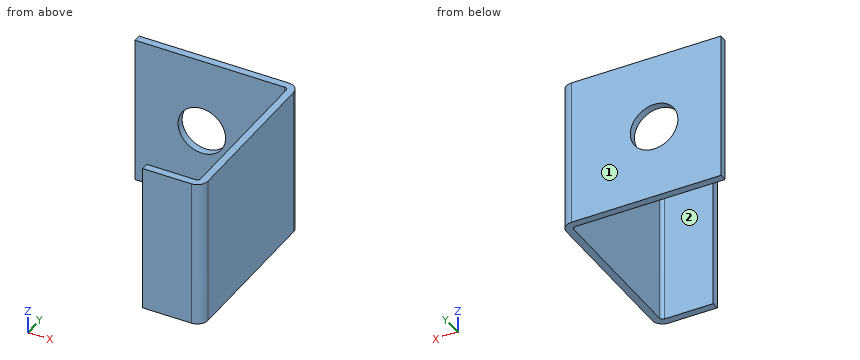
```python
from build123d import *

# Parameters (mm, degrees)
SKETCH1_W                     = 32.7025
SKETCH1_H                     = 31.75
SKETCH1_R                     = 5.08
HV_FUSE_BASE_DEPTH            = 1.5875
FUSE_TO_STACK_STRIP_W         = 7.8232
FUSE_TO_STACK_STRIP_H         = 1.5875
FUSE_TO_STACK_STRIP_CUT_DEPTH = 31.75
FUSE_TO_STACK_DEPTH           = 31.75
STACK_BASE_STRIP_W            = 7.8232
STACK_BASE_STRIP_H            = 1.5875
STACK_BASE_STRIP_CUT_DEPTH    = 31.75
STACK_BASE_DEPTH              = 31.75


# Sheet-metal steps are written as plain solids
with BuildPart() as part:
    # Sketch1 → HV Fuse Base (new body)
    with BuildSketch(Plane(origin=(0, 0, 0), x_dir=(1, 0, 0), z_dir=(0, 1, 0))):
        with Locations((16.35125, -15.875)):
            Rectangle(SKETCH1_W, SKETCH1_H)
        with Locations(Location((14.2875, -15.875, 0), (0, 0, 270))):
            Circle(SKETCH1_R, mode=Mode.SUBTRACT)
    extrude(amount=-HV_FUSE_BASE_DEPTH)

    # Fuse to Stack strip (across the edge) → Fuse to Stack strip cut (cut)
    with BuildSketch(Plane(origin=(32.7025, -1.5875, 0), x_dir=(-1, 0, 0), z_dir=(0, 0, 1))):
        with Locations((-3.175, -0.79375)):
            Rectangle(FUSE_TO_STACK_STRIP_W, FUSE_TO_STACK_STRIP_H)
    extrude(amount=FUSE_TO_STACK_STRIP_CUT_DEPTH, mode=Mode.SUBTRACT)

    # Fuse to Stack section (across the edge) → Fuse to Stack (add)
    with BuildSketch(Plane(origin=(32.7025, -1.5875, 0), x_dir=(-1, 0, 0), z_dir=(0, 0, 1))):
        with BuildLine():
            Line((-1.5875, 0.7366), (-1.5875, 36.22802))
            Line((-1.5875, 36.22802), (0, 36.22802))
            Line((0, 36.22802), (0, 0.7366))
            ThreePointArc((0, 0.7366), (0.215745145, 0.215745145), (0.7366, 0))
            Line((0.7366, 0), (0.7366, -1.5875))
            ThreePointArc((0.7366, -1.5875), (-0.90678687, -0.90678687), (-1.5875, 0.7366))
        make_face()
    extrude(amount=FUSE_TO_STACK_DEPTH)

    # Stack Base strip (across the edge) → Stack Base strip cut (cut)
    with BuildSketch(Plane(origin=(32.7025, -37.81552, 0), x_dir=(0, 1, 0), z_dir=(0, 0, 1))):
        with Locations((-1.5875, -0.79375)):
            Rectangle(STACK_BASE_STRIP_W, STACK_BASE_STRIP_H)
    extrude(amount=STACK_BASE_STRIP_CUT_DEPTH, mode=Mode.SUBTRACT)

    # Stack Base section (across the edge) → Stack Base (add)
    with BuildSketch(Plane(origin=(32.7025, -37.81552, 0), x_dir=(0, 1, 0), z_dir=(0, 0, 1))):
        with BuildLine():
            Line((0, 0.7366), (0, 11.1125))
            Line((0, 11.1125), (1.5875, 11.1125))
            Line((1.5875, 11.1125), (1.5875, 0.7366))
            ThreePointArc((1.5875, 0.7366), (1.803245145, 0.215745145), (2.3241, 0))
            Line((2.3241, 0), (2.3241, -1.5875))
            ThreePointArc((2.3241, -1.5875), (0.68071313, -0.90678687), (0, 0.7366))
        make_face()
    extrude(amount=STACK_BASE_DEPTH)


solid = part.part
```
Verification items for the finished model (mm, model axes). Face numbers are marked on the shaded views. A direction names the side the tool comes from. Give positions to 0.01 mm unless a question says otherwise; leave off trailing zeros. Order: outer loops, then holes, each group sorted by start corner. A loop starts at its lowest first (then second) coordinate and runs counter-clockwise, first axis right, second up. Notation, with made-up numbers: M -4,10.25 L 27,10.25 A14 ccw 27,15.25 Z; hole C 33.25,24.5 d3. An arc over 180 degrees is marked long. Return JSON: item names as keys, results as strings. Group by question number.
1) Go/stop test with flat-tipped pins: pin 1 Ø1.5 at (y, z) = (-12.5, 5.5) entering from -X; pin 2 Ø6 at (x, y) = (28, -33) entering from +Z; pin 3 Ø11.5 at (x, z) = (14.29, 15.88) entering from -Y; pin 4 Ø1.7 at (y, z) = (-37, 13.5) entering from -X. Record where each tip stops, or that it passes through.
2) Section check B-B on z = 24. Record the cut outline in (x, y), and give its area (3 significant figures).
3) Access from +Z, -Z, +X, -X, +Y, -Y to the whole of each face (thin tool, end or side, straight path). Record for the marked faces 1 and 2.
4) Section check C-C on x = 13. Record the cut outline in (y, z), and give its area (3 significant figures).
5) Section check A-A on x = 29.5. Record the cut outline in (y, z), and give its area (3 significant figures).
6) Scan lines: line 1 (Y direction, x = 23, z = 14); line 2 (Y direction, x = 4.5, z = 18.5); line 3 (X direction, y = -30, z = 21). Record each from-to range of solid material in increasing order.
7) Section check D-D on z = 20. Record the cut outline in (x, y), and give its area (3 significant figures).
Answer block:
{
 "1": {"pin 1": "stops at x = 32.7", "pin 2": "passes through", "pin 3": "stops at y = -1.59", "pin 4": "stops at x = 21.59"},
 "2": {"outline": "M 0,-1.59 L 31.97,-1.59 A0.74 cw 32.7,-2.32 L 32.7,-35.49 A0.74 cw 31.97,-36.23 L 21.59,-36.23 L 21.59,-37.82 L 31.97,-37.82 A2.32 ccw 34.29,-35.49 L 34.29,-2.32 A2.32 ccw 31.97,0 L 0,0 Z", "area": "128 mm^2"},
 "3": {"face 1": "+Z, -Z, +X, -X, +Y", "face 2": "+Z, -Z, -X"},
 "4": {"outline": "M -1.59,0 L 0,0 L 0,10.96 L -1.59,10.96 Z; M -1.59,20.79 L 0,20.79 L 0,31.75 L -1.59,31.75 Z", "area": "34.8 mm^2"},
 "5": {"outline": "M -37.82,0 L -36.23,0 L -36.23,31.75 L -37.82,31.75 Z; M -1.59,0 L 0,0 L 0,31.75 L -1.59,31.75 Z", "area": "101 mm^2"},
 "6": {"line 1": "y = -37.82 to -36.23, -1.59 to 0", "line 2": "y = -1.59 to 0", "line 3": "x = 32.7 to 34.29"},
 "7": {"outline": "M 0,-1.59 L 11.32,-1.59 L 11.32,0 L 0,0 Z; M 17.25,-1.59 L 31.97,-1.59 A0.74 cw 32.7,-2.32 L 32.7,-35.49 A0.74 cw 31.97,-36.23 L 21.59,-36.23 L 21.59,-37.82 L 31.97,-37.82 A2.32 ccw 34.29,-35.49 L 34.29,-2.32 A2.32 ccw 31.97,0 L 17.25,0 Z", "area": "118 mm^2"}
}
